Build history of the part. All positions in model axes, mm. A direction names the side the tool comes from. Give positions to 0.01 mm unless a question says otherwise; leave off trailing zeros. Order: outer loops, then holes, each group sorted by start corner. A loop starts at its lowest first (then second) coordinate and runs counter-clockwise, first axis right, second up. Notation, with made-up numbers: (76, -38) - (111, -38) arc R23 ccw to (111, -28) - close; hole circle Ø1 at (-23, 72). An arc over 180 degrees is marked (long way). Use a Markdown table: item, result. Add a question column.
(1) Flat gauge pins, fed straight in: pin 1 (4 mm diameter, centred on x = -38.5, z = 3, fed in from +Y); pin 2 (2 mm diameter, centred on y = 16.5, z = 2.5, fed in from -X); pin 3 (4 mm diameter, centred on x = 42.5, z = 3, fed in from -Y); pin 4 (12 mm diameter, centred on x = 42, y = 19.5, fed in from -Z). Where does each tip first touch, or does it go through?
(2) Slice it at C-C (y = 21.5). Write the cut outline in (x, z).
(3) Slice it at D-D (x = 36). Write the cut outline in (y, z), then the cut area to 3 significant figures.
(4) Slice it at A-A (y = -1.5). Count the separate pieces of the cut face and the enclosed holes in it, then the cut area to 3 significant figures.
(5) Slice it at B-B (x = 12). Write the cut outline in (y, z).
(6) Wall check: line 1 (Z direction, x = 55, y = 3.75); line 2 (Y direction, x = -28.5, z = 2.75); line 3 (X direction, y = 17, z = 2.75). Give the ranges that are in metal, low to high.
(7) Which spindle directions (+Z, -Z, +X, -X, +Y, -Y) get a long thin tool onto all of the face, cutting with end or side? Do faces 4 (the face through (1, 0, 8)), 5 (the face through (-39, 12.5, 4)), 6 (the face through (-20, -18, 4)), 7 (the face through (20, 18, 4)). Say none if no direction does.
(8) Mould opens along X. For faces 1 (the face through (1, 0, 0)), 2 (the face through (11.425, 0.35, 5.386)), 3 (the face through (19, -24, 4)) say: +X half, -X half, draft (parallel to the pull), parting line (faces both ways), or undercut.
from build123d import *

# Parameters (mm, degrees)
EXTRUDE_1_DEPTH     = 8
CHAMFER_1_SIZE      = 2
SKETCH_4_R          = 1.5
CUT_EXTRUDE_3_DEPTH = 50
CHAMFER_3_SIZE      = 2
FILLET_1_R          = 4
SKETCH_6_R          = 1.5
CUT_EXTRUDE_5_DEPTH = 72.205687975


with BuildPart() as part:
    # 草图1 → 凸台-拉伸1 (new body)
    with BuildSketch(Plane.XY):
        Polygon((-20, 25), (20, 25), (20, 12.5), (60, 12.5), (60, -12.5), (20, -12.5), (20, -25), (-20, -25), (-20, -12.5), (-60, -12.5), (-60, 12.5), (-20, 12.5), align=None)
    extrude(amount=EXTRUDE_1_DEPTH)

    # 倒角1
    chamfer_1_edges = [part.edges().sort_by_distance(p)[0] for p in [
        (20, -25, 4),
        (-20, -25, 4),
        (-20, 25, 4),
        (20, 25, 4),
    ]]
    chamfer(chamfer_1_edges, length=CHAMFER_1_SIZE)

    # 草图4 → 切除-拉伸3 (cut)
    with BuildSketch(Plane(origin=(0, 25, 0), x_dir=(1, 0, 0), z_dir=(0, 1, 0))):
        with Locations(Location((-12, -4, 0), (0, 0, 270))):
            Circle(SKETCH_4_R)
        with Locations(Location((0, -4, 0), (0, 0, 270))):
            Circle(SKETCH_4_R)
        with Locations(Location((12, -4, 0), (0, 0, 270))):
            Circle(SKETCH_4_R)
    extrude(amount=-CUT_EXTRUDE_3_DEPTH, mode=Mode.SUBTRACT)

    # 倒角3
    chamfer_3_edges = [part.edges().sort_by_distance(p)[0] for p in [
        (-60, -12.5, 4),
        (-60, 12.5, 4),
        (60, 12.5, 4),
        (60, -12.5, 4),
    ]]
    chamfer(chamfer_3_edges, length=CHAMFER_3_SIZE)

    # 圆角1
    fillet_1_edges = [part.edges().sort_by_distance(p)[0] for p in [
        (60, 0, 0),
        (60, 0, 8),
        (-60, 0, 0),
        (-60, 0, 8),
    ]]
    fillet(fillet_1_edges, radius=FILLET_1_R - 0.0001)  # a hair under: the kernel refuses the full size

    # 草图6 → 切除-拉伸5 (cut, through all)
    with BuildSketch(Plane(origin=(0, 12.5, 0), x_dir=(1, 0, 0), z_dir=(0, 1, 0))):
        with Locations(Location((55, -4, 0), (0, 0, 180))):
            Circle(SKETCH_6_R)
    cut_extrude_5 = extrude(amount=-CUT_EXTRUDE_5_DEPTH, mode=Mode.SUBTRACT)

    # 镜向4: 切除-拉伸5 across plane
    add(cut_extrude_5.mirror(Plane(origin=(0, 0, 0), x_dir=(0, 0, 1), z_dir=(1, 0, 0))), mode=Mode.SUBTRACT)


solid = part.part
Solution:
| question | item | result |
|---|---|---|
| 1 | pin 1 | y = 12.5 |
| 1 | pin 2 | x = -20 |
| 1 | pin 3 | y = -12.5 |
| 1 | pin 4 | through |
| 2 | outline | (-20, 0) - (20, 0) - (20, 8) - (-20, 8) - close; hole circle Ø3 at (-12, 4); hole circle Ø3 at (0, 4); hole circle Ø3 at (12, 4) |
| 3 | outline | (-12.5, 0) - (12.5, 0) - (12.5, 8) - (-12.5, 8) - close |
| 3 | area | 200 mm2 |
| 4 | separate pieces | 1 |
| 4 | enclosed holes | 5 |
| 4 | area | 911 mm2 |
| 5 | outline | (-25, 0) - (25, 0) - (25, 2.5) - (-25, 2.5) - close; (-25, 5.5) - (25, 5.5) - (25, 8) - (-25, 8) - close |
| 6 | line 1 | 0 to 2.5, 5.5 to 8 |
| 6 | line 2 | -12.5 to 12.5 |
| 6 | line 3 | -20 to -12.83, -11.17 to -0.83, 0.83 to 11.17, 12.83 to 20 |
| 7 | face 4 | +Z, +X, -X, +Y, -Y |
| 7 | face 5 | +Z, -Z, -X, +Y |
| 7 | face 6 | +Z, -Z, -X, -Y |
| 7 | face 7 | +Z, -Z, +X, +Y |
| 8 | face 1 | draft |
| 8 | face 2 | undercut |
| 8 | face 3 | +X half |
